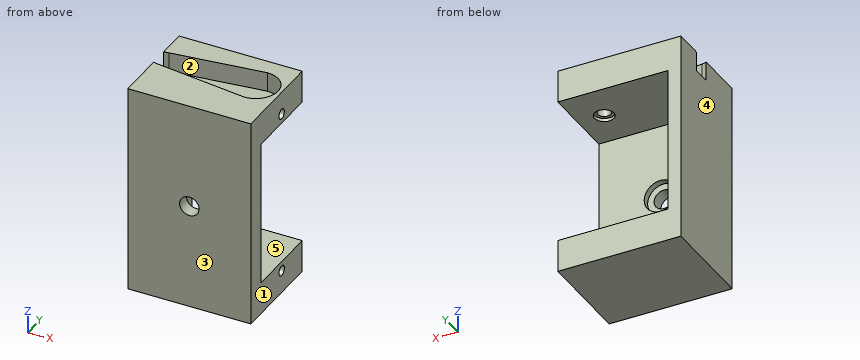
from build123d import *

# Parameters (mm, degrees)
SKETCH_1_W           = 5
SKETCH_1_H           = 12
EXTRUDE_1_DEPTH      = 19
EXTRUDE_1_2_DEPTH    = 19
SKETCH_2_W           = 32.5
SKETCH_2_H           = 12
EXTRUDE_2_DEPTH      = 2
SKETCH_3_R           = 0.785
CUT_EXTRUDE_2_DEPTH  = 3
CUT_EXTRUDE_3_DEPTH  = 3
EXTRUDE_START        = 1
SKETCH_7_R           = 0.785
EXTRUDE_3_DEPTH      = 1
SKETCH_8_W           = 4.508312044
SKETCH_8_H           = 2.561477722
SKETCH_8_R           = 1
CUT_EXTRUDE_9_DEPTH  = 1
SKETCH_9_R           = 1
CUT_EXTRUDE_10_DEPTH = 3
SKETCH_12_R          = 1.5
CUT_EXTRUDE_11_DEPTH = 0.5
SKETCH_13_W          = 19
SKETCH_13_H          = 32.5
EXTRUDE_4_DEPTH      = 3
SKETCH_14_R          = 1.5
CUT_EXTRUDE_12_DEPTH = 3
SKETCH_15_R          = 2.5
CUT_EXTRUDE_13_DEPTH = 1


with BuildPart() as part:
    # Sketch 1 → Extrude 1 (new body)
    with BuildSketch(Plane(origin=(0, 0, 0), x_dir=(0, 0, -1), z_dir=(1, 0, 0))):
        with Locations((-13.75, 0)):
            Rectangle(SKETCH_1_W, SKETCH_1_H)
    extrude(amount=EXTRUDE_1_DEPTH)



with BuildPart() as body_2:
    # Sketch 1 → Extrude 1 2 (new body)
    with BuildSketch(Plane(origin=(0, 0, 0), x_dir=(0, 0, -1), z_dir=(1, 0, 0))):
        with Locations((13.75, 0)):
            Rectangle(SKETCH_1_W, SKETCH_1_H)
    extrude(amount=EXTRUDE_1_2_DEPTH)


with BuildPart() as part_1:
    add(part.part)

    add(body_2.part)  # Extrude 2 merges body 2
    # Sketch 2 → Extrude 2 (add)
    with BuildSketch(Plane.ZY):
        Rectangle(SKETCH_2_W, SKETCH_2_H)
    extrude(amount=-EXTRUDE_2_DEPTH)

    # Sketch 3 → Cut-Extrude 2 (cut)
    with BuildSketch(Plane(origin=(19, 0, 0), x_dir=(0, 0, -1), z_dir=(1, 0, 0))):
        with Locations((-12.72, 0)):
            Circle(SKETCH_3_R)
        with Locations((12.72, 0)):
            Circle(SKETCH_3_R)
    extrude(amount=-CUT_EXTRUDE_2_DEPTH, mode=Mode.SUBTRACT)

    # Sketch 4 → Cut-Extrude 3 (cut)
    with BuildSketch(Plane.XY.offset(16.25)):
        with BuildLine():
            ThreePointArc((0.75, 1.6), (-0.85, 0), (0.75, -1.6))
            Line((0.75, -1.6), (15, -3.45))
            ThreePointArc((15, -3.45), (18.45, 0), (15, 3.45))
            Line((15, 3.45), (0.75, 1.6))
        make_face()
    extrude(amount=-CUT_EXTRUDE_3_DEPTH, mode=Mode.SUBTRACT)

    # Sketch 7 → Extrude 3 (add)
    with BuildSketch(Plane(origin=(16, 0, 0), x_dir=(0, 0, -1), z_dir=(1, 0, 0)).offset(EXTRUDE_START)):
        with Locations((-12.72, 0)):
            Circle(SKETCH_7_R)
    extrude(amount=-EXTRUDE_3_DEPTH)

    # Sketch 8 → Cut-Extrude 9 (cut)
    with BuildSketch(Plane.XY.offset(13.25)):
        with Locations((15, 0)):
            Rectangle(SKETCH_8_W, SKETCH_8_H)
        with Locations((15, 0)):
            Circle(SKETCH_8_R, mode=Mode.SUBTRACT)
    extrude(amount=CUT_EXTRUDE_9_DEPTH, mode=Mode.SUBTRACT)

    # Sketch 9 → Cut-Extrude 10 (cut)
    with BuildSketch(Plane.XY.offset(13.25)):
        with Locations((15, 0)):
            Circle(SKETCH_9_R)
    extrude(amount=-CUT_EXTRUDE_10_DEPTH, mode=Mode.SUBTRACT)

    # Sketch 12 → Cut-Extrude 11 (cut)
    with BuildSketch(Plane(origin=(0, 0, 11.25), x_dir=(-1, 0, 0), z_dir=(0, 0, -1))):
        with Locations((-15, 0)):
            Circle(SKETCH_12_R)
    extrude(amount=-CUT_EXTRUDE_11_DEPTH, mode=Mode.SUBTRACT)

    # Sketch 13 → Extrude 4 (add)
    with BuildSketch(Plane.XZ.offset(6)):
        with Locations((9.5, 0)):
            Rectangle(SKETCH_13_W, SKETCH_13_H)
    extrude(amount=EXTRUDE_4_DEPTH)

    # Sketch 14 → Cut-Extrude 12 (cut)
    with BuildSketch(Plane.XZ.offset(9)):
        with Locations(Location((9.5, 0, 0), (0, 0, 270))):
            Circle(SKETCH_14_R)
    extrude(amount=-CUT_EXTRUDE_12_DEPTH, mode=Mode.SUBTRACT)

    # Sketch 15 → Cut-Extrude 13 (cut)
    with BuildSketch(Plane(origin=(0, -6, 0), x_dir=(1, 0, 0), z_dir=(0, 1, 0))):
        with Locations(Location((9.5, 0, 0), (0, 0, 270))):
            Circle(SKETCH_15_R)
    extrude(amount=-CUT_EXTRUDE_13_DEPTH, mode=Mode.SUBTRACT)


solid = part_1.part
Could you check a few things on this model? Use its own coordinates, in mm. Face numbers are marked on the shaded views. A direction names the side the tool comes from. Coordinates: 2 decimals unless noted, no trailing zeros. Order: outer loops, then holes, each group sorted by start corner. A loop starts at its lowest first (then second) coordinate and runs counter-clockwise, first axis right, second up. Notation, with made-up numbers: (23.5, 48.25) -> (79.5, 48.25) arc R26 ccw to (79.5, 76.25) -> close; hole circle Ø4 at (-14, 14.25). An arc over 180 degrees is marked (long way). One line per question, with ' | ' between items.
Q1. I'm going to push flat-ended pins straight in: P1, Ø4, axis at x = 9.5, z = 0, coming from the +Y side; P2, Ø1.5, axis at y = -1.5, z = -7, coming from the +X side; P3, Ø1.5, axis at x = 5, y = -1, coming from the +Z side. Where does each tip first touch, or does it pass through?
Return value:
P1: y = -7 | P2: x = 2 | P3: z = 13.25
Q2. On a 3-axis mill with a long thin cutter (end or side, diameter ignored), from which of +Z, -Z, +X, -X, +Y, -Y can I reach the whole of each face in a straight line? I mean the marked faces 4 and 5. Say none if no direction works.
Return value:
face 4: +Z, -Z, -X, +Y, -Y | face 5: +X, +Y
Q3. Imagine slicing it at A-A on z = 12.72. Please give me the cut outline in (x, y) (3 decimals).
Return value:
outline: (0, -9) -> (19, -9) -> (19, -0.785) -> (17, -0.785) -> (17, 0.785) -> (19, 0.785) -> (19, 6) -> (0, 6) -> close; hole circle Ø2 at (15, 0)
Q4. Thinking about a two-plate mould opening in X: for the marked faces 1, 2 and 3, which applies, pulls with the +X half, pulls with the -X half, needs draft (parallel to the pull), parting line crosses it, or undercut?
Return value:
face 1: pulls with the +X half | face 2: undercut | face 3: needs draft
Q5. If I drill on L1, parallel to Y at x = 15, z = 12.35; L2, parallel to Z at x = 17.5, y = 2.5; L3, parallel to Y at x = 16.9, z = -12.72 (3 decimals), over which ranges is the centre line in solid material (lowest first)?
Return value:
L1: -9 to -1, 1 to 6 | L2: -16.25 to -11.25, 11.25 to 16.25 | L3: -9 to -0.785, 0.785 to 6
Q6. Imagine slicing it at C-C on z = 0. Please give me the cut outline in (x, y), and give its area (3 significant figures).
Return value:
outline: (0, -9) -> (8, -9) -> (8, -7) -> (7, -7) -> (7, -6) -> (2, -6) -> (2, 6) -> (0, 6) -> close; (11, -9) -> (19, -9) -> (19, -6) -> (12, -6) -> (12, -7) -> (11, -7) -> close | area: 70.0 mm²
Q7. Imagine slicing it at B-B on y = 0. Please give me the cut outline in (x, z) (3 decimals).
Return value:
outline: (0, -16.25) -> (19, -16.25) -> (19, -13.505) -> (16, -13.505) -> (16, -11.935) -> (19, -11.935) -> (19, -11.25) -> (2, -11.25) -> (2, 11.25) -> (13.5, 11.25) -> (13.5, 11.75) -> (14, 11.75) -> (14, 13.25) -> (0, 13.25) -> close; (16, 11.75) -> (16.5, 11.75) -> (16.5, 11.25) -> (19, 11.25) -> (19, 11.935) -> (17, 11.935) -> (17, 13.25) -> (16, 13.25) -> close; (18.45, 13.505) -> (19, 13.505) -> (19, 16.25) -> (18.45, 16.25) -> close
Q8. Imagine slicing it at D-D on x = 9.5. Please give me the cut outline in (y, z), and give its area (3 significant figures).
Return value:
outline: (-9, -16.25) -> (6, -16.25) -> (6, -11.25) -> (-6, -11.25) -> (-6, -2.5) -> (-7, -2.5) -> (-7, -1.5) -> (-9, -1.5) -> close; (-9, 1.5) -> (-7, 1.5) -> (-7, 2.5) -> (-6, 2.5) -> (-6, 11.25) -> (6, 11.25) -> (6, 16.25) -> (2.74, 16.25) -> (2.74, 13.25) -> (-2.74, 13.25) -> (-2.74, 16.25) -> (-9, 16.25) -> close | area: 190 mm²
